Geometry check sheet. Reference: the model listing, model coordinates, mm. Face numbers are marked on the shaded views. A direction names the side the tool comes from. Coordinates: 2 decimals unless noted, no trailing zeros. Loops run counter-clockwise (first coordinate to the right, second up) from the corner with the lowest first, then second, coordinate; pieces in that order, holes last. Notation, with made-up numbers: (-2.75, 43) - (53.25, 43) arc R33 cw to (53.25, 73) - close; hole circle Ø10 at (-20.5, 2). An arc over 180 degrees is marked (long way). Write each question's results on one line, items separated by ' | '. Start each with the question number.
(1) Material ranges on probe 1 along X at (y, z) = (12.5, 1.15); probe 2 along Y at (x, z) = (2.15, 0.45); probe 3 along Y at (x, z) = (3.65, 0.15), recorded low to high.
(2) Mould release check, pull along Y, two halves, no side actions. Record for the marked faces 1 and 2: pulls with the +Y half, pulls with the -Y half, needs draft (parallel to the pull), parting line crosses it, or undercut.
(3) Sectioned sample at B-B (z = 0.5). Enter the section's corners in (x, y), plus the area to 3 significant figures.
(4) Sectioned sample at C-C (y = 32). Enter the section's corners in (x, z), plus the area to 3 significant figures.
(5) Sectioned sample at A-A (x = 3.2). Enter the section's corners in (y, z), plus the area to 3 significant figures.
(6) Access from +Z, -Z, +X, -X, +Y, -Y to the whole of each face (thin tool, end or side, straight path). Record for the marked faces 3 and 4.
from build123d import *

# Parameters (mm, degrees)
BOSS_EXTRUDE1_DEPTH = 2
BOSS_EXTRUDE2_DEPTH = 4


with BuildPart() as part:
    # Sketch1 → Boss-Extrude1 (new body)
    with BuildSketch(Plane.YZ):
        with BuildLine():
            ThreePointArc((0, 1.5), (-0.75, 0.75), (0, 0))
            Line((0, 0), (0, 1.5))
        make_face()
        with BuildLine():
            Line((0, 1.5), (0, 0))
            ThreePointArc((0, 0), (0.530330086, 0.219669914), (0.75, 0.75))
            ThreePointArc((0.75, 0.75), (0.530330086, 1.280330086), (0, 1.5))
        make_face()
        with BuildLine():
            ThreePointArc((0.75, 0.75), (0.530330086, 0.219669914), (0, 0))
            Line((0, 0), (37, 0))
            ThreePointArc((37, 0), (36.25, 0.75), (37, 1.5))
            Line((37, 1.5), (0, 1.5))
            ThreePointArc((0, 1.5), (0.530330086, 1.280330086), (0.75, 0.75))
        make_face()
        with BuildLine():
            ThreePointArc((37, 1.5), (36.25, 0.75), (37, 0))
            Line((37, 0), (37, 1.5))
        make_face()
        with BuildLine():
            Line((37, 1.5), (37, 0))
            ThreePointArc((37, 0), (37.530330086, 0.219669914), (37.75, 0.75))
            ThreePointArc((37.75, 0.75), (37.530330086, 1.280330086), (37, 1.5))
        make_face()
    extrude(amount=BOSS_EXTRUDE1_DEPTH)

    # Sketch1_3 → Boss-Extrude2 (add)
    with BuildSketch(Plane.YZ):
        with BuildLine():
            ThreePointArc((37, 1.5), (36.25, 0.75), (37, 0))
            Line((37, 0), (37, 1.5))
        make_face()
        with BuildLine():
            Line((37, 1.5), (37, 0))
            ThreePointArc((37, 0), (37.530330086, 0.219669914), (37.75, 0.75))
            ThreePointArc((37.75, 0.75), (37.530330086, 1.280330086), (37, 1.5))
        make_face()
        with BuildLine():
            ThreePointArc((0, 1.5), (-0.75, 0.75), (0, 0))
            Line((0, 0), (0, 1.5))
        make_face()
        with BuildLine():
            Line((0, 1.5), (0, 0))
            ThreePointArc((0, 0), (0.530330086, 0.219669914), (0.75, 0.75))
            ThreePointArc((0.75, 0.75), (0.530330086, 1.280330086), (0, 1.5))
        make_face()
    extrude(amount=BOSS_EXTRUDE2_DEPTH)


solid = part.part
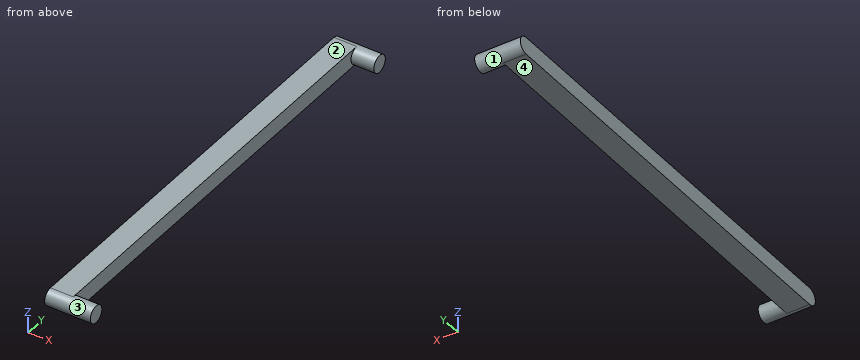
Outcome:
1) probe 1: x = 0 to 2 | probe 2: y = -0.69 to 0.69, 36.31 to 37.69 | probe 3: y = -0.45 to 0.45, 36.55 to 37.45
2) face 1: undercut | face 2: needs draft
3) outline: (0, -0.71) - (4, -0.71) - (4, 0.71) - (2, 0.71) - (2, 36.29) - (4, 36.29) - (4, 37.71) - (0, 37.71) - close | area: 82.5 mm2
4) outline: (0, 0) - (2, 0) - (2, 1.5) - (0, 1.5) - close | area: 3.00 mm2
5) outline: circle Ø1.5 at (0, 0.75); circle Ø1.5 at (37, 0.75) | area: 3.53 mm2
6) face 3: +X | face 4: -Z, +X, -X, +Y, -Y
